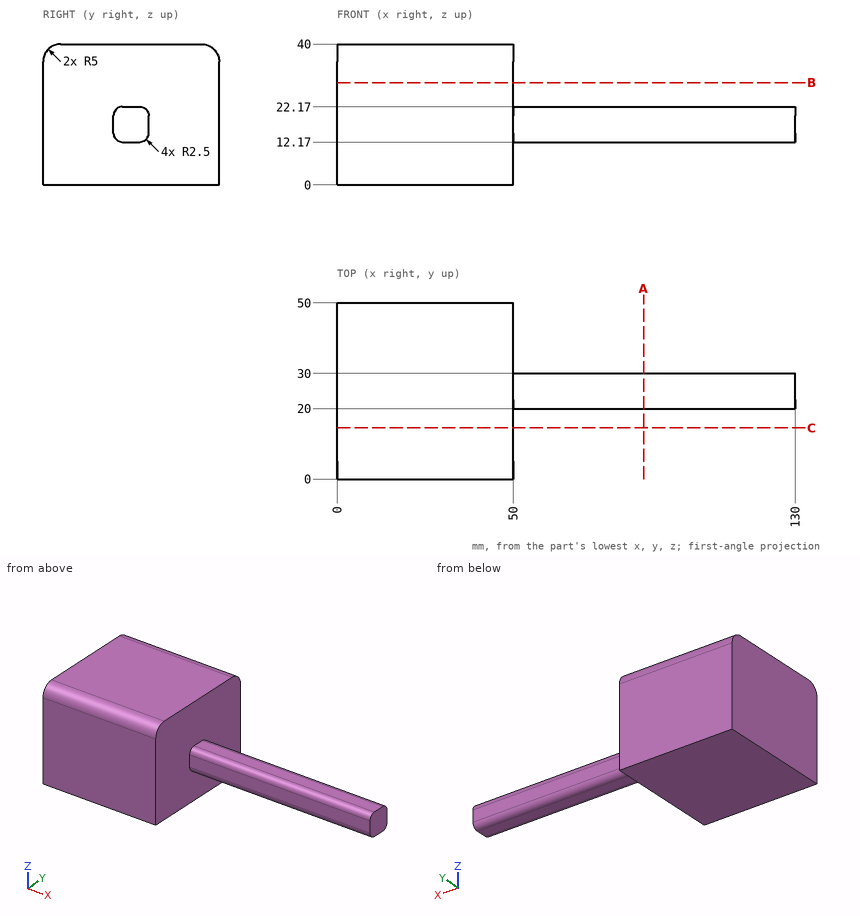
Part print with two shaded views. Sizes in mm from the minimum x, y, z corner. Round coordinates to 2 decimals unless told otherwise and drop trailing zeros. Order: outer loops, then holes, each group sorted by start corner. A loop starts at its lowest first (then second) coordinate and runs counter-clockwise, first axis right, second up. Notation, with made-up numbers: (-3.5, -30) - (50.5, -30) arc R17 ccw to (50.5, -13) - close; hole circle Ø10 at (16, -9.75). An arc over 180 degrees is marked (long way). Answer in a Markdown table with one row per item. Add a question column.
(1) Band-saw the part on C-C on y = 14.5. List the corners of the cut face in (x, z).
(2) Drop flat-ended pins along their axis: pin 1 Ø4 at (x, y) = (79, 24.5) entering from -Z; pin 2 Ø1 at (y, z) = (41.5, 8) entering from +X; pin 3 Ø5.5 at (x, z) = (99, 17) entering from +Y. Give the stop position or say it passes through.
(3) Band-saw the part on B-B on z = 29. List the corners of the cut face in (x, y).
(4) Probe L1, parallel to X at y = 45.5, z = 34.5; L2, parallel to Z at x = 123.5, y = 25; L3, parallel to Y at x = 59, z = 17.5. List the from-to ranges inside material, lowest first. Write a range as [from, to].
(5) Band-saw the part on A-A on x = 87. List the corners of the cut face in (y, z).
Data:
| question | item | result |
|---|---|---|
| 1 | outline | (0, 0) - (50, 0) - (50, 40) - (0, 40) - close |
| 2 | pin 1 | stops at z = 12.17 |
| 2 | pin 2 | stops at x = 50 |
| 2 | pin 3 | stops at y = 30 |
| 3 | outline | (0, 0) - (50, 0) - (50, 50) - (0, 50) - close |
| 4 | L1 | x = [0, 50] |
| 4 | L2 | z = [12.17, 22.17] |
| 4 | L3 | y = [20, 30] |
| 5 | outline | (20, 14.67) arc R2.5 ccw to (22.5, 12.17) - (27.5, 12.17) arc R2.5 ccw to (30, 14.67) - (30, 19.67) arc R2.5 ccw to (27.5, 22.17) - (22.5, 22.17) arc R2.5 ccw to (20, 19.67) - close |
